For this review, take the finished solid that the model builds, in its own axes (mm). A direction names the side the tool comes from. Round coordinates to 2 decimals unless told otherwise and drop trailing zeros. Order: outer loops, then holes, each group sorted by start corner. A loop starts at its lowest first (then second) coordinate and runs counter-clockwise, first axis right, second up. Notation, with made-up numbers: (47, 31.25) -> (68, 31.25) arc R22 cw to (68, 53.25) -> close; hole circle Ø2 at (80, 56.5). An arc over 180 degrees is marked (long way). Use a Markdown table: item, result. Add a question column.
1) Clearance check with flat-ended pins moving along their axes: P1, Ø6, axis at x = 2.5, y = 20, coming from the +Z side; P2, Ø7.5, axis at x = 15, y = 6.5, coming from the +Z side; P3, Ø5, axis at x = 13, y = 11, coming from the +Z side. State where each tip first meets the part, or that it passes through.
2) Consider section A-A (x = 12). State the section outline as (y, z) points, plus the area to 3 significant figures.
3) Machinability: for faces 1 (the face through (15.001, 19, -15)), 2 (the face through (13, 0, -22)), 3 (the face through (7, 12.7, -13)), which of the approach directions +Z, -Z, +X, -X, +Y, -Y give a long, thin tool a straight path to every point of the face, cutting with its end or side? Answer none if there is none.
4) Wall thickness on line 1 along Z through (x, y) = (7.75, 7); line 2 along Y through (x, z) = (9, -9.25); line 3 along Z through (x, y) = (1.75, 21): over which ranges is each line inside the solid? List them lowest first. Write a range as [from, to].
5) Consider section D-D (x = 2). State the section outline as (y, z) points.
6) Consider section B-B (z = -8.25). State the section outline as (x, y) points, plus the area to 3 significant figures.
7) Consider section C-C (y = 23). State the section outline as (x, z) points, plus the area to 3 significant figures.
```python
from build123d import *

# Parameters (mm, degrees)
F0_W      = 25.4
F0_H      = 38.1
F1_DEPTH  = 25.4
F2_W      = 25.4
F2_H      = 19.05
F3_DEPTH  = 12.7
F5_DEPTH  = 25.4
F6_W      = 25.4
F6_H      = 12.7
F7_DEPTH  = 25.4
F8_W      = 6.35
F8_H      = 4.064
F9_DEPTH  = 25.4
F11_DEPTH = 25.4


with BuildPart() as f1:
    # F0 (on Top) → F1 (new body)
    with BuildSketch(Plane.XY):
        with Locations((12.7, 19.05)):
            Rectangle(F0_W, F0_H)
    extrude(amount=-F1_DEPTH)

    # F2 (on Front) → F3 (cut)
    with BuildSketch(Plane.XZ):
        with Locations((12.7, -9.525)):
            Rectangle(F2_W, F2_H)
    extrude(amount=-F3_DEPTH, mode=Mode.SUBTRACT)

    # F4 (on face) → F5 (cut)
    with BuildSketch(Plane.XZ.offset(-12.7)):
        Polygon((25.4, 0), (0, 0), (25.4, -19.05), align=None)
    extrude(amount=-F5_DEPTH, mode=Mode.SUBTRACT)

    # F6 (on Top) → F7 (join)
    with BuildSketch(Plane.XY):
        with Locations((12.7, 19.05)):
            Rectangle(F6_W, F6_H)
    extrude(amount=-F7_DEPTH)

    # F8 (on Front) → F9 (cut)
    with BuildSketch(Plane.XZ):
        with Locations((3.175, -2.032)):
            Rectangle(F8_W, F8_H)
    extrude(amount=-F9_DEPTH, mode=Mode.SUBTRACT)

    # F10 (on Front) → F11 (cut)
    with BuildSketch(Plane.XZ):
        Polygon((15.000969, 0), (15.000969, -11.250727), (15.000969, -19.05), (27.700969, -19.05), (27.700969, 0), align=None)
        Polygon((15.000969, 0), (0, 0), (15.000969, -11.250727), align=None)
    extrude(amount=-F11_DEPTH, mode=Mode.SUBTRACT)


solid = f1.part
```
Results list:
| question | item | result |
|---|---|---|
| 1 | P1 | z = -4.06 |
| 1 | P2 | z = -19.05 |
| 1 | P3 | z = -8.38 |
| 2 | outline | (0, -25.4) -> (38.1, -25.4) -> (38.1, -9) -> (12.7, -9) -> (12.7, -19.05) -> (0, -19.05) -> close |
| 2 | area | 497 mm2 |
| 3 | face 1 | +Z, +X, -Y |
| 3 | face 2 | +Z, -Z, +X, -X, -Y |
| 3 | face 3 | +Z, +X, -X, -Y |
| 4 | line 1 | [-25.4, -19.05] |
| 4 | line 2 | [12.7, 38.1] |
| 4 | line 3 | [-25.4, -4.06] |
| 5 | outline | (0, -25.4) -> (38.1, -25.4) -> (38.1, -1.5) -> (25.4, -1.5) -> (25.4, -4.06) -> (12.7, -4.06) -> (12.7, -19.05) -> (0, -19.05) -> close |
| 6 | outline | (0, 12.7) -> (11, 12.7) -> (11, 38.1) -> (0, 38.1) -> close |
| 6 | area | 279 mm2 |
| 7 | outline | (0, -25.4) -> (25.4, -25.4) -> (25.4, -19.05) -> (15, -19.05) -> (15, -11.25) -> (5.42, -4.06) -> (0, -4.06) -> close |
| 7 | area | 352 mm2 |
